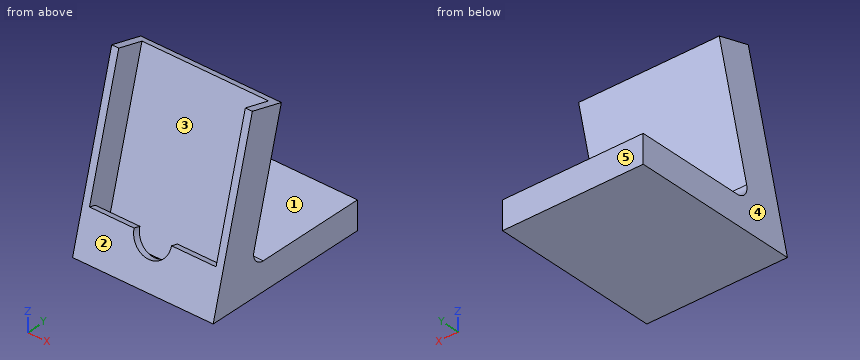
from build123d import *

# Parameters (mm, degrees)
F1_DEPTH = 63.5
F2_W     = 57.15
F2_H     = 9.525
F3_DEPTH = 72.39
F5_DEPTH = 3.175
F6_R     = 5.08


with BuildPart() as f1:
    # F0 (on Right) → F1 (new body)
    with BuildSketch(Plane.YZ):
        Polygon((20.6850513497, 77.1976625943), (0, 0), (76.2, 0), (76.2, 12.7), (19.8379641079, 12.7), (36.0191238421, 73.0889102533), align=None)
    extrude(amount=F1_DEPTH)

    # F2 (on face) → F3 (cut)
    with BuildSketch(Plane(origin=(0, 20.6850513497, 77.1976625943), x_dir=(1, 0, 0), z_dir=(0, 0.2588190451, 0.9659258263))):
        with Locations((31.75, 7.9375)):
            Rectangle(F2_W, F2_H)
    extrude(amount=-F3_DEPTH, mode=Mode.SUBTRACT)

    # F4 (on face) → F5 (cut, through all)
    with BuildSketch(Plane(origin=(0, 0, 0), x_dir=(1, 0, 0), z_dir=(0, -0.9659258263, 0.2588190451))):
        Polygon((60.325, 79.9209012672), (3.175, 79.9209012672), (3.175, 20.2309012672), (23.2833333333, 20.2309012672), (40.2166666667, 20.2309012672), (60.325, 20.2309012672), align=None)
        with BuildLine():
            Line((40.2166666667, 20.2309012672), (23.2833333333, 20.2309012672))
            ThreePointArc((23.2833333333, 20.2309012672), (31.75, 11.7642346006), (40.2166666667, 20.2309012672))
        make_face()
    extrude(amount=-F5_DEPTH, mode=Mode.SUBTRACT)

    # F6
    f6_edges = [f1.edges().sort_by_distance(p)[0] for p in [
        (31.75, 19.837964, 12.7),
    ]]
    fillet(f6_edges, radius=F6_R)


solid = f1.part
The model under review builds one solid part; all positions refer to its coordinate system, in mm. Face numbers are marked on the shaded views. A direction names the side the tool comes from. Round coordinates to 2 decimals unless told otherwise and drop trailing zeros. Loops run counter-clockwise (first coordinate to the right, second up) from the corner with the lowest first, then second, coordinate; pieces in that order, holes last. Notation, with made-up numbers: (35.5, -11) -> (87.5, -11) arc R12 cw to (87.5, 0) -> close; hole circle Ø1 at (79.25, 6). An arc over 180 degrees is marked (long way). One line per question, with ' | ' between items. Start each with the question number.
Item 1: Add section D-D, the plane x = 28. Write out the cut boundary in (y, z), then the cut area to 3 significant figures.
Item 2: Add section B-B, the plane z = 63.5. Write out the cut boundary in (x, y) (3 decimals), then the cut area to 3 significant figures.
Item 3: Add section C-C, the plane y = 16.5. Write out the cut boundary in (x, z) (3 decimals), then the cut area to 3 significant figures.
Item 4: Add section A-A, the plane x = 11. Write out the cut boundary in (y, z).
Item 5: Machinability: for the marked faces 1 and 2, which of the approach directions +Z, -Z, +X, -X, +Y, -Y give a long, thin tool a straight path to every point of the face, cutting with its end or side? Answer none if there is none.
Item 6: Wall thickness on line 1 along Z through (x, y) = (22.5, 60.5); line 2 along X through (y, z) = (25, 51) (3 decimals); line 3 along Y through (x, z) = (12.5, 32): over which ranges is each line inside the solid? List them lowest first. Write a range as [from, to].
Item 7: Draft analysis for pull direction X (two halves, no side actions). For the marked faces 3, 4 and 5, state which applies: +X half, -X half, draft (parallel to the pull), parting line (faces both ways), or undercut.
Item 8: For pin 1 (10 mm diameter, centred on x = 8, y = 42.5, fed in from +Z); pin 2 (4 mm diameter, centred on x = 7, z = 22.5, fed in from -Y); pin 3 (12 mm diameter, centred on x = 9, y = 24.5, fed in from +Z), all flat-tipped, find the tip position at first contact; note any pin that passes through.
Return value:
1) outline: (0, 0) -> (76.2, 0) -> (76.2, 12.7) -> (26.46, 12.7) arc R5.08 cw to (21.55, 19.09) -> (36.02, 73.09) -> (32.95, 73.91) -> (14.22, 3.99) -> (5.02, 6.45) -> (6.34, 11.39) -> (3.27, 12.21) -> close | area: 1,080 mm2
2) outline: (0, 17.015) -> (3.175, 17.015) -> (3.175, 30.163) -> (60.325, 30.163) -> (60.325, 17.015) -> (63.5, 17.015) -> (63.5, 33.45) -> (0, 33.45) -> close | area: 292 mm2
3) outline: (0, 0) -> (63.5, 0) -> (63.5, 61.579) -> (60.325, 61.579) -> (60.325, 12.51) -> (3.175, 12.51) -> (3.175, 61.579) -> (0, 61.579) -> close | area: 1,110 mm2
4) outline: (0, 0) -> (76.2, 0) -> (76.2, 12.7) -> (26.46, 12.7) arc R5.08 cw to (21.55, 19.09) -> (36.02, 73.09) -> (32.95, 73.91) -> (14.22, 3.99) -> (5.02, 6.45) -> (8.3, 18.72) -> (5.24, 19.54) -> close
5) face 1: +X, -X, +Y | face 2: +Z, +X, -X, -Y
6) line 1: z = [0, 12.7] | line 2: x = [0, 3.175], [60.325, 63.5] | line 3: y = [21.72, 25.01]
7) face 3: undercut | face 4: -X half | face 5: draft
8) pin 1: stops at z = 12.7 | pin 2: stops at y = 18.64 | pin 3: stops at z = 76.56
